Input: part model. Units: mm. Frame: model coordinates. Coordinates: 2 decimals unless noted, no trailing zeros. Write each loop counter-clockwise with the first axis right and the second up, starting at its lowest first coordinate (ties: lowest second). Pieces come first, ordered by that corner, then holes.
Autodesk Inventor part; units mm, degrees
ref_plane "YZ Plane" through (0, 0, 0) normal (1, 0, 0) x (0, 1, 0)
ref_plane "XZ Plane" through (0, 0, 0) normal (0, 1, 0) x (-1, 0, 0)
ref_plane "XY Plane" through (0, 0, 0) normal (0, 0, 1) x (1, 0, 0)
sketch "Boceto39" plane through (0, 0, 0) normal (0, 0, 1) x (1, 0, 0)
  line L0 (-18.25, 4.75) -> (18.25, 4.75)
  line L1 (18.25, 4.75) -> (18.25, -4.75)
  line L2 (18.25, -4.75) -> (-18.25, -4.75)
  line L3 (-18.25, -4.75) -> (-18.25, 4.75)
  point P0 (0, 0)
  point P1 (0, 4.75)
  point P2 (-18.25, 0)
  dimension "d373" = 36.5
  dimension "d374" = 9.5
extrude "Extrusión13" add sketch "Boceto39" along normal blind 9.5
sketch "Boceto40" plane through (0, 0, 0) normal (0, 1, 0) x (-1, 0, 0)
  line L0 (18.25, 0) -> (-18.25, 0)
  line L1 (18.25, 0) -> (18.25, 9.5)
  line L2 (-18.25, 9.5) -> (18.25, 9.5)
  line L3 (-18.25, 0) -> (-18.25, 9.5)
  line L4 (-20, -4.2347) -> (-20, 2.75)
  line L5 (-18, 4.75) -> (18, 4.75)
  line L6 (20, 2.75) -> (20, -6)
  arc A0 (20, 2.75) -> (18, 4.75) centre (18, 2.75) ccw
  arc A1 (-18, 4.75) -> (-20, 2.75) centre (-18, 2.75) ccw
  point P0 (0, 0)
  point P1 (0, 4.75)
  point P2 (18.25, 4.75)
  point P3 (0, 0)
  dimension "d377" = 20
  dimension "d378" = 2
  dimension "d379" = 6
sketch "Boceto41" plane through (0, 0, 0) normal (1, 0, 0) x (0, 1, 0)
  circle A0 centre (0, 4.75) radius 0.4
  point P0 (0, 0)
  dimension "d380" = 0.8
sweep "Barrido1" add profiles "Boceto41" path "Boceto40" path curves L6 A0 L5 A1 L4
properties part number "AXIAL-POWER-10W"
Item 1: Section query D-D, the plane z = -5. Return loops of the section in (x, y).
Item 2: Material intervals for line 1 (Z direction, x = -1.5, y = -1.5); line 2 (X direction, y = -3, z = 5.5), sorted ascending.
Item 3: Pin query (flat end, axial travel): pin 1 Ø1 at (x, y) = (16, 1) entering from -Z; pin 2 Ø0.6 at (x, y) = (20, 0) entering from -Z; pin 3 Ø4 at (y, z) = (-3.5, 6.5) entering from -X. Return the tip coordinate at first contact, or that it passes through.
Item 4: Section query C-C, the plane y = 0. Return loops of the section in (x, z), then the cut area to 3 significant figures.
Item 5: Section query B-B, the plane z = -1.5. Return loops of the section in (x, y).
Item 6: Section query A-A, the plane z = 1.75. Return loops of the section in (x, y), then the cut area to 3 significant figures.
The answers:
1. outline: circle Ø0.8 at (-20, 0)
2. line 1: z = 0 to 9.5
2. line 2: x = -18.25 to 18.25
3. pin 1: stops at z = 0
3. pin 2: stops at z = -4.23
3. pin 3: stops at x = -18.25
4. outline: (-20.4, -6) - (-19.6, -6) - (-19.6, 2.75) arc R1.6 cw to (-18.25, 4.33) - (-18.25, 0) - (18.25, 0) - (18.25, 4.33) arc R1.6 cw to (19.6, 2.75) - (19.6, -4.23) - (20.4, -4.23) - (20.4, 2.75) arc R2.4 ccw to (18.25, 5.14) - (18.25, 9.5) - (-18.25, 9.5) - (-18.25, 5.14) arc R2.4 ccw to (-20.4, 2.75) - close
4. area: 364 mm2
5. outline: circle Ø0.8 at (-20, 0); circle Ø0.8 at (20, 0)
6. outline: circle Ø0.8 at (-20, 0); (-18.25, -4.75) - (18.25, -4.75) - (18.25, 4.75) - (-18.25, 4.75) - close; circle Ø0.8 at (20, 0)
6. area: 348 mm2
